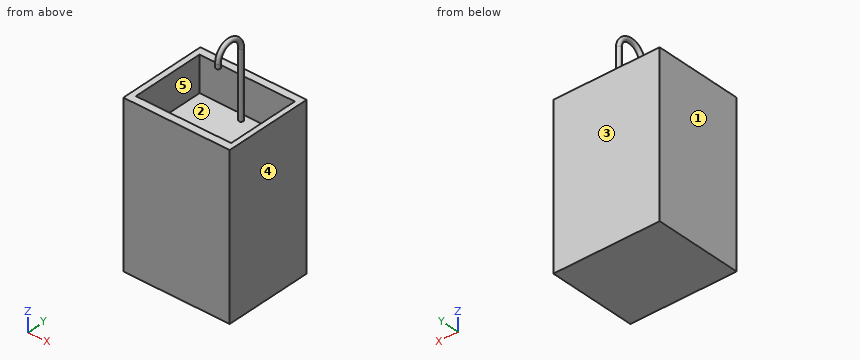
from build123d import *

# Parameters (mm, degrees)
F0_W     = 600
F0_H     = 500
F1_DEPTH = 900
F2_W     = 537.3239591718
F2_H     = 413.3979640901
F3_DEPTH = 200
F6_R     = 12.5


# Not quite as in the source:
# - a feature names something its author has since deleted; it is built from what else it names


with BuildPart() as f1:
    # F0 (on Top) → F1 (new body)
    with BuildSketch(Plane.XY):
        with Locations((300, 250)):
            Rectangle(F0_W, F0_H)
    extrude(amount=F1_DEPTH)

    # F2 (on face) → F3 (cut)
    with BuildSketch(Plane.XY.offset(900)):
        with Locations((301.7210625112, 250.2208668739)):
            Rectangle(F2_W, F2_H)
    extrude(amount=-F3_DEPTH, mode=Mode.SUBTRACT)

    # F7: sweep along a path in F5
    with BuildLine(Plane(origin=(300, 0, 0), x_dir=(0, -1, 0), z_dir=(-1, 0, 0))) as f7_path:
        Line((-420, 589.8187315079), (-420, 1075))
        ThreePointArc((-420, 1075), (-398.033008589, 1128.033008589), (-345, 1150))
        ThreePointArc((-345, 1150), (-291.966991411, 1128.033008589), (-270, 1075))
        Line((-270, 1075), (-270, 1050))
    # F6 (on face) → F7 (sweep)
    with BuildSketch(Plane.XY.offset(700)):
        with Locations((300.0000119209, 420.0000464916)):
            Circle(F6_R)
    sweep(path=f7_path.line)


solid = f1.part
Work out the finished part from the listing and answer in its coordinate system (mm). Face numbers are marked on the shaded views. A direction names the side the tool comes from. Give positions to 0.01 mm unless a question says otherwise; leave off trailing zeros. Write each loop counter-clockwise with the first axis right and the second up, starting at its lowest first coordinate (ties: lowest second). Pieces come first, ordered by that corner, then holes.
Q1. Straight lines are drawn through the part: L1, parallel to X at y = 440.5, z = 804; L2, parallel to Z at x = 143, y = 95; L3, parallel to Z at x = 102, y = 38. For each, find the intervals that lie inside material, in ascending order.
Answer:
L1: x = 0 to 33.06, 570.38 to 600
L2: z = 0 to 700
L3: z = 0 to 900
Q2. A tool of negligible diameter and unlimited length cuts with its end or side. For the marked faces 4 and 5, from which of +Z, -Z, +X, -X, +Y, -Y can it reach the whole face along a straight path? Write none if from no direction.
Answer:
face 4: +Z, -Z, +X, +Y, -Y
face 5: +Z
Q3. The part is cut by section A-A on x = 364. Give the vertices of the cut face in (y, z).
Answer:
outline: (0, 0) - (500, 0) - (500, 900) - (456.92, 900) - (456.92, 700) - (43.52, 700) - (43.52, 900) - (0, 900) - close
Q4. The part is cut by section B-B on y = 84. Give the vertices of the cut face in (x, z).
Answer:
outline: (0, 0) - (600, 0) - (600, 900) - (570.38, 900) - (570.38, 700) - (33.06, 700) - (33.06, 900) - (0, 900) - close
Q5. The part is cut by section C-C on z = 847. Give the vertices of the cut face in (x, y).
Answer:
outline: (0, 0) - (600, 0) - (600, 500) - (0, 500) - close; circle Ø25 at (300, 420); hole (33.06, 43.52) - (570.38, 43.52) - (570.38, 456.92) - (33.06, 456.92) - close
Q6. Given pin 1 (1.5 mm diameter, centred on x = 538, y = 159, fed in from +Z), flat-ended and moving along its own axis, determine where the tip first touches the part or whether it passes through.
Answer:
pin 1: stops at z = 700
Q7. For a pull along X with two mould halves and no side action, classify the marked faces 1, 2 and 3 as released by +X, released by -X, zero draft, split by the parting line, or undercut.
Answer:
face 1: released by -X
face 2: undercut
face 3: zero draft
